The listing builds one solid part. Answer for the finished solid, in the listing's coordinates (mm). Face numbers are marked on the shaded views. A direction names the side the tool comes from. Round coordinates to 2 decimals unless told otherwise and drop trailing zeros. Loops run counter-clockwise (first coordinate to the right, second up) from the corner with the lowest first, then second, coordinate; pieces in that order, holes last. Notation, with made-up numbers: (30.25, 20.5) - (88.25, 20.5) arc R9 ccw to (88.25, 27.5) - close; hole circle Ø8 at (89.25, 30). An arc over 180 degrees is marked (long way). One line per question, with ' | ' between items. Start each with the question number.
from build123d import *

# Parameters (mm, degrees)
F1_DEPTH = 6
F3_DEPTH = 7.001
F4_R     = 4.75
F5_DEPTH = 25


with BuildPart() as f1:
    # F0 (on Front) → F1 (new body, symmetric)
    with BuildSketch(Plane.XZ):
        Polygon((7, 25), (0, 25), (0, 0), (25, 0), (25, 7), (7, 7), align=None)
    extrude(amount=F1_DEPTH, both=True)

    # F2 (on face) → F3 (cut, through all)
    with BuildSketch(Plane.XY.offset(7)):
        with BuildLine():
            ThreePointArc((25, -3.68273), (26.290251, -2.038688), (26.75, 0))
            ThreePointArc((26.75, 0), (26.290251, 2.038688), (25, 3.68273))
            Line((25, 3.68273), (25, -3.68273))
        make_face()
        with BuildLine():
            Line((25, -3.68273), (25, 3.68273))
            ThreePointArc((25, 3.68273), (17.25, 0), (25, -3.68273))
        make_face()
    extrude(amount=-F3_DEPTH, mode=Mode.SUBTRACT)

    # F4 (on face) → F5 (cut)
    with BuildSketch(Plane.YZ.offset(7)):
        with Locations((0, 22)):
            Circle(F4_R)
    extrude(amount=-F5_DEPTH, mode=Mode.SUBTRACT)


solid = f1.part
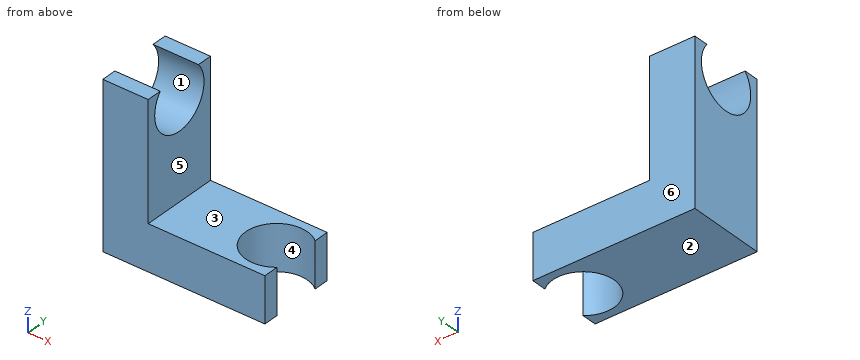
(1) Find section D-D on y = 0.5. Write down the section's boundary in (x, z).
(2) Each of these flat-tipped pins is pushed along its axis until it touches: P1, Ø2, axis at x = 11, y = 2.5, coming from the +Z side; P2, Ø6, axis at y = -1, z = 16, coming from the +X side. Where does it stop, or does it pass through?
(3) Consider L1, parallel to Y at x = 22, z = 2.25; L2, parallel to Z at x = 15.75, y = 5. Determine where each line is inside the solid, lowest interval first.
(4) Find section C-C on y = 4.25. Write down the section's boundary in (x, z).
(5) A tool of negligible diameter and unlimited length cuts with its end or side. For the marked faces 5 and 6, from which of +Z, -Z, +X, -X, +Y, -Y can it reach the whole face along a straight path? Write none if from no direction.
(6) Determine the mould class of the marked faces 1, 2, 3 and 4 for opening direction Z: pulls with the +Z half, pulls with the -Z half, needs draft (parallel to the pull), parting line crosses it, or undercut.
(7) Find section B-B on z = 22. Write down the section's boundary in (x, y).
(8) Find section A-A on x = 22. Write down the section's boundary in (y, z), plus the area to 3 significant figures.
Answer below:
1) outline: (0, 0) - (17.28, 0) - (17.28, 7) - (7, 7) - (7, 17.28) - (0, 17.28) - close
2) P1: z = 7 | P2: x = 7
3) L1: -6 to -4.75, 4.75 to 6 | L2: 0 to 7
4) outline: (0, 0) - (19.88, 0) - (19.88, 7) - (7, 7) - (7, 19.88) - (0, 19.88) - close; (0, 24.12) - (7, 24.12) - (7, 25) - (0, 25) - close; (24.12, 0) - (25, 0) - (25, 7) - (24.12, 7) - close
5) face 5: +Z, +X, +Y, -Y | face 6: +Z, -Z, +X, -X, +Y
6) face 1: undercut | face 2: pulls with the -Z half | face 3: pulls with the +Z half | face 4: needs draft
7) outline: (0, -6) - (7, -6) - (7, -4.75) - (0, -4.75) - close; (0, 4.75) - (7, 4.75) - (7, 6) - (0, 6) - close
8) outline: (-6, 0) - (-4.75, 0) - (-4.75, 7) - (-6, 7) - close; (4.75, 0) - (6, 0) - (6, 7) - (4.75, 7) - close | area: 17.5 mm2
